Part model, mm, in its own coordinate system. A direction names the side the tool comes from. Round coordinates to 2 decimals unless told otherwise and drop trailing zeros. Loops run counter-clockwise (first coordinate to the right, second up) from the corner with the lowest first, then second, coordinate; pieces in that order, holes last.
1) 3-axis set-ups, long thin cutter, end or side, ignore diameter. For faces 1 (the cylindrical face through (6.018, -2.495, 8.049)), 2 (the flat face through (-103, -43, 19.05)): which of +Z, -Z, +X, -X, +Y, -Y reach the whole face in a straight line?
2) Band-saw the part on D-D, the plane z = 31. State how many separate pieces and enclosed holes the cut face has, then the cut area to 3 significant figures.
3) Band-saw the part on B-B, the plane y = 101.6. Write the cut outline in (x, z) (3 decimals).
4) Probe line 1 (Y direction, x = -127, z = 31); line 2 (X direction, y = -12, z = 22); line 3 (X direction, y = -46, z = 30). List the from-to ranges inside material, lowest first.
5) Band-saw the part on A-A, the plane x = 0. Write the cut outline in (y, z) (3 decimals), then the cut area to 3 significant figures.
6) Mould opens along X. For faces 3 (the flat face through (152.4, -2, 19)), 4 (the flat face through (-2, -152.4, 19)), 5 (the flat face through (55, -80, 19.05)) say: +X half, -X half, draft (parallel to the pull), parting line (faces both ways), or undercut.
7) Band-saw the part on C-C, the plane x = -127. Write the cut outline in (y, z) (3 decimals).
8) Drop flat-ended pins along their axis: P1, Ø2.5, axis at x = -69, y = -41.5, coming from the +Z side; P2, Ø3.5, axis at x = -41.5, y = 28.5, coming from the +Z side. Give the stop position or say it passes through.
from build123d import *

# Parameters (mm, degrees)
SKETCH1_W                = 304.8
SKETCH1_H                = 304.8
BOSS_EXTRUDE1_DEPTH      = 38.1
SKETCH2_R                = 6.5151
HAAS_T_SLOT_HOLES_DEPTH  = 219.867836833
SKETCH3_R                = 9.779
HAAS_COUNTER_BORES_DEPTH = 22.225
SKETCH4_R                = 3.2639
CUT_EXTRUDE1_DEPTH       = 19.05
SKETCH5_R                = 2.414626773
SKETCH5_R_2              = 2.5
CUT_EXTRUDE2_DEPTH       = 12.7


with BuildPart() as part:
    # Sketch1 → Boss-Extrude1 (new body)
    with BuildSketch(Plane.XY):
        Rectangle(SKETCH1_W, SKETCH1_H)
    extrude(amount=BOSS_EXTRUDE1_DEPTH)

    # Sketch2 → HAAS T-Slot Holes (cut, through all)
    with BuildSketch(Plane.XY.offset(38.1)):
        with Locations((-127, 101.6)):
            Circle(SKETCH2_R)
        with Locations((127, 101.6)):
            Circle(SKETCH2_R)
        with Locations((127, -101.6)):
            Circle(SKETCH2_R)
        with Locations((-127, -101.6)):
            Circle(SKETCH2_R)
        Circle(SKETCH2_R)
    extrude(amount=-HAAS_T_SLOT_HOLES_DEPTH, mode=Mode.SUBTRACT)

    # Sketch3 → HAAS Counter Bores (cut)
    with BuildSketch(Plane.XY.offset(38.1)):
        with Locations((-127, 101.6)):
            Circle(SKETCH3_R)
        with Locations((127, 101.6)):
            Circle(SKETCH3_R)
        Circle(SKETCH3_R)
        with Locations((127, -101.6)):
            Circle(SKETCH3_R)
        with Locations((-127, -101.6)):
            Circle(SKETCH3_R)
    extrude(amount=-HAAS_COUNTER_BORES_DEPTH, mode=Mode.SUBTRACT)

    # Sketch4 → Cut-Extrude1 (cut)
    with BuildSketch(Plane.XY.offset(38.1)):
        with Locations((55.338636384, -31.78626265)):
            Circle(SKETCH4_R)
        with Locations((-103.268864702, -43.062839234)):
            Circle(SKETCH4_R)
        with Locations((-41.984915865, -11.846060915)):
            Circle(SKETCH4_R)
        with Locations((-41.984915865, 28.793939085)):
            Circle(SKETCH4_R)
        with Locations((123.115084135, 27.523939085)):
            Circle(SKETCH4_R)
        with Locations((-137.234915865, -80.426060915)):
            Circle(SKETCH4_R)
        with Locations((55.514563309, -80.426060915)):
            Circle(SKETCH4_R)
        with Locations((33.602258032, 57.632075165)):
            Circle(SKETCH4_R)
        with Locations((57.786056257, 56.797137583)):
            Circle(SKETCH4_R)
    extrude(amount=-CUT_EXTRUDE1_DEPTH, mode=Mode.SUBTRACT)

    # Sketch5 → Cut-Extrude2 (cut)
    with BuildSketch(Plane.XY.offset(38.1)):
        with Locations((-41.984915865, 65.623939085)):
            Circle(SKETCH5_R)
        with Locations((-92.209313854, 35.743562234)):
            Circle(SKETCH5_R_2)
        with Locations((-69.254539014, -41.750458903)):
            Circle(SKETCH5_R_2)
        with Locations((15.165084135, 8.473939085)):
            Circle(SKETCH5_R_2)
    extrude(amount=-CUT_EXTRUDE2_DEPTH, mode=Mode.SUBTRACT)


solid = part.part
Reported:
1. face 1: +Z, -Z
1. face 2: +Z
2. separate pieces: 1
2. enclosed holes: 18
2. area: 91,000 mm2
3. outline: (-152.4, 0) - (-133.515, 0) - (-133.515, 15.875) - (-136.779, 15.875) - (-136.779, 38.1) - (-152.4, 38.1) - close; (-120.485, 0) - (120.485, 0) - (120.485, 15.875) - (117.221, 15.875) - (117.221, 38.1) - (-117.221, 38.1) - (-117.221, 15.875) - (-120.485, 15.875) - close; (133.515, 0) - (152.4, 0) - (152.4, 38.1) - (136.779, 38.1) - (136.779, 15.875) - (133.515, 15.875) - close
4. line 1: y = -152.4 to -111.38, -91.82 to 91.82, 111.38 to 152.4
4. line 2: x = -152.4 to -45.25, -38.72 to 152.4
4. line 3: x = -152.4 to -104.69, -101.85 to 152.4
5. outline: (-152.4, 0) - (-6.515, 0) - (-6.515, 15.875) - (-9.779, 15.875) - (-9.779, 38.1) - (-152.4, 38.1) - close; (6.515, 0) - (152.4, 0) - (152.4, 38.1) - (9.779, 38.1) - (9.779, 15.875) - (6.515, 15.875) - close
5. area: 11,000 mm2
6. face 3: +X half
6. face 4: draft
6. face 5: undercut
7. outline: (-152.4, 0) - (-108.115, 0) - (-108.115, 15.875) - (-111.379, 15.875) - (-111.379, 38.1) - (-152.4, 38.1) - close; (-95.085, 0) - (95.085, 0) - (95.085, 15.875) - (91.821, 15.875) - (91.821, 38.1) - (-91.821, 38.1) - (-91.821, 15.875) - (-95.085, 15.875) - close; (108.115, 0) - (152.4, 0) - (152.4, 38.1) - (111.379, 38.1) - (111.379, 15.875) - (108.115, 15.875) - close
8. P1: stops at z = 25.4
8. P2: stops at z = 19.05
